For this review, take the finished solid that the model builds, in its own axes (mm). Coordinates: 2 decimals unless noted, no trailing zeros. Return JSON: item names as keys, results as strings. Group by question number.
Item 1: Insertion check: pin 1 (1.5 mm diameter, centred on x = 0, y = -64, fed in from +Z). The pin has a flat end and moves straight along its axis. Give the tip position at first contact, or say it passes through.
Item 2: For line 1 along Z through (x, y) = (-7.5, 232); line 2 along Z through (x, y) = (0, -58.5); line 3 along Z through (x, y) = (-9, 246.5), list the stretches that pass through material, from the lowest coordinate up.
Item 3: Take a section at A-A (y = -16). Count the separate pieces of the cut face and the enclosed holes in it, then the cut area to 3 significant figures.
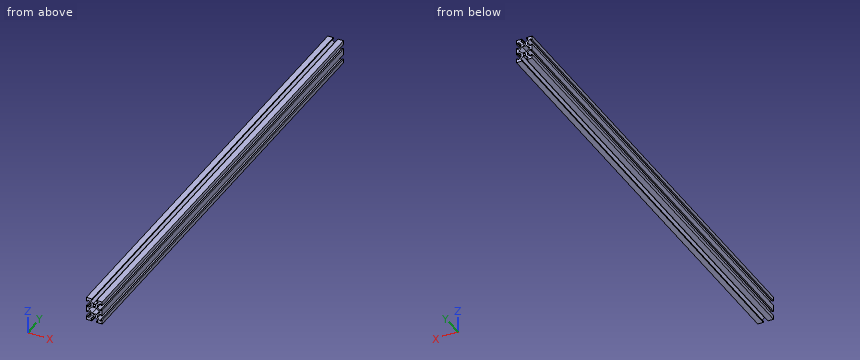
```python
from build123d import *

# Parameters (mm, degrees)
SKETCH_R  = 1.5
PAD_DEPTH = 290


with BuildPart() as part:
    # Sketch → Pad (new body, symmetric)
    with BuildSketch(Plane.XZ):
        Polygon((-10, 30), (-3, 30), (-3, 28.5), (-4.5, 28.5), (-4.5, 27), (-1.5, 24), (1.5, 24), (4.5, 27), (4.5, 28.5), (3, 28.5), (3, 30), (10, 30), (10, 25), (8.5, 25), (8.5, 26.5), (7, 26.5), (4, 23.5), (4, 20.5), (7, 17.5), (8.5, 17.5), (8.5, 19), (10, 19), (10, 11), (8.5, 11), (8.5, 12.5), (7, 12.5), (4, 9.5), (4, 6.5), (7, 3.5), (8.5, 3.5), (8.5, 5), (10, 5), (10, 0), (3, 0), (3, 1.5), (4.5, 1.5), (4.5, 3), (1.5, 6), (-1.5, 6), (-4.5, 3), (-4.5, 1.5), (-3, 1.5), (-3, 0), (-10, 0), (-10, 5), (-8.5, 5), (-8.5, 3.5), (-7, 3.5), (-4, 6.5), (-4, 9.5), (-7, 12.5), (-8.5, 12.5), (-8.5, 11), (-10, 11), (-10, 19), (-8.5, 19), (-8.5, 17.5), (-7, 17.5), (-4, 20.5), (-4, 23.5), (-7, 26.5), (-8.5, 26.5), (-8.5, 25), (-10, 25), align=None)
        with Locations((0, 8)):
            Circle(SKETCH_R, mode=Mode.SUBTRACT)
        with Locations((0, 22)):
            Circle(SKETCH_R, mode=Mode.SUBTRACT)
        Polygon((-7, 15), (-2.716354, 19.283646), (2.716354, 19.283646), (7, 15), (2.716354, 10.716354), (-2.716354, 10.716354), align=None, mode=Mode.SUBTRACT)
    extrude(amount=PAD_DEPTH, both=True)


solid = part.part
```
Findings below:
{
 "1": {"pin 1": "stops at z = 24"},
 "2": {"line 1": "z = 0 to 3.5, 12.5 to 17.5, 26.5 to 30", "line 2": "z = 6 to 6.5, 9.5 to 10.72, 19.28 to 20.5, 23.5 to 24", "line 3": "z = 0 to 5, 11 to 19, 25 to 30"},
 "3": {"separate pieces": "1", "enclosed holes": "3", "area": "260 mm2"}
}
